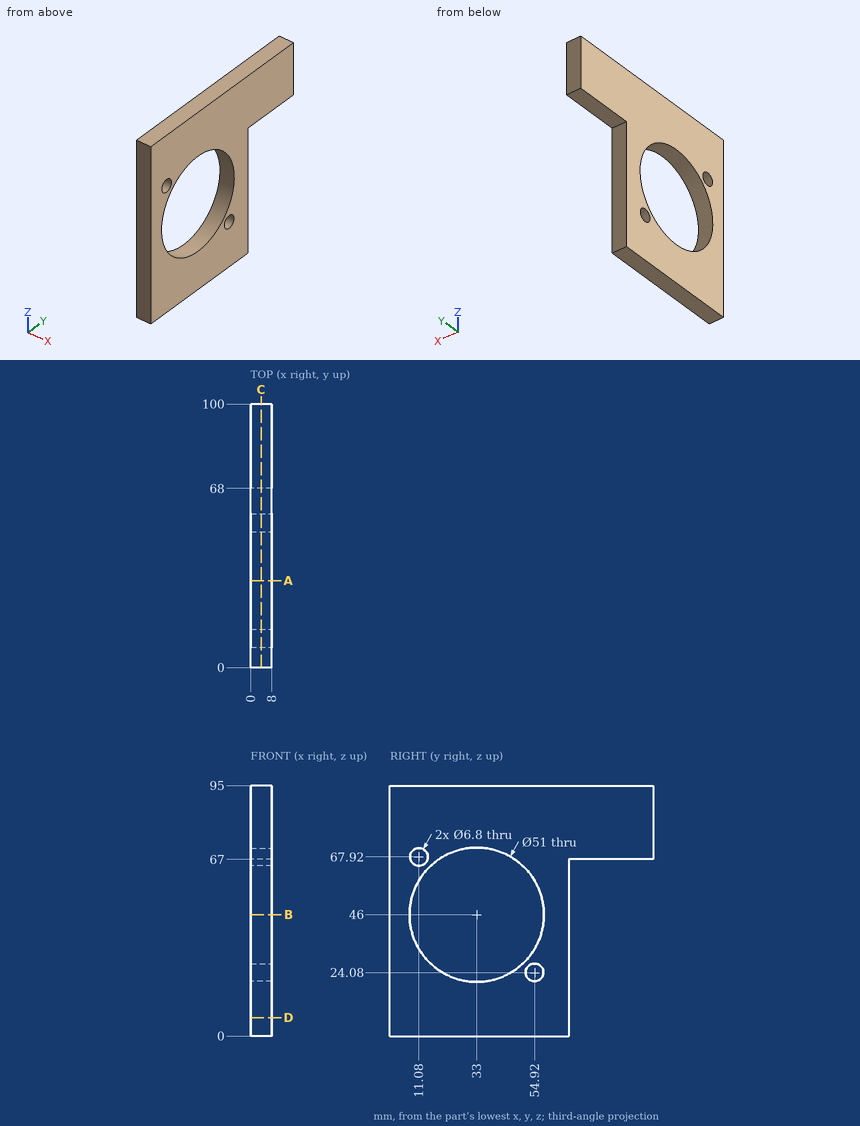
The drawing under review shows one solid part. Ordinate dimensions are in mm from its lowest x, y, z. Give positions to 0.01 mm unless a question says otherwise; leave off trailing zeros. Write each loop counter-clockwise with the first axis right and the second up, starting at its lowest first coordinate (ties: lowest second). Pieces come first, ordered by that corner, then holes. Notation, with made-up numbers: (73.25, 84.5) -> (77.25, 84.5) arc R21 ccw to (77.25, 97.5) -> close; hole circle Ø10 at (23.5, 10). An arc over 180 degrees is marked (long way). Use CSV: the item, a comma, the result in double quotes.
Q1. For P1, Ø4, axis at x = 3.5, y = 86, coming from the -Z side, flat-tipped, find the tip position at first contact; note if it passes through.
Conclusion:
P1,"z = 67"
Q2. Take a section at D-D, the plane z = 7. Write out the cut boundary in (x, y).
Conclusion:
outline,"(0, 0) -> (8, 0) -> (8, 68) -> (0, 68) -> close"
Q3. To check wall thickness, follow probe 1 along Z at (x, y) = (5.5, 55.5); probe 2 along Y at (x, z) = (2.5, 46); probe 3 along Y at (x, z) = (7.5, 27) (1 decimal). State the ranges of each line that lie inside material, in increasing order. Write a range as [from, to].
Conclusion:
probe 1,"[0, 20.73], [27.43, 34], [58, 95]"
probe 2,"[0, 7.5], [58.5, 68]"
probe 3,"[0, 16], [50, 53.2], [56.7, 68]"
Q4. Take a section at B-B, the plane z = 46. Write out the cut boundary in (x, y).
Conclusion:
outline,"(0, 0) -> (8, 0) -> (8, 7.5) -> (0, 7.5) -> close; (0, 58.5) -> (8, 58.5) -> (8, 68) -> (0, 68) -> close"
Q5. Take a section at C-C, the plane x = 4. Write out the cut boundary in (y, z).
Conclusion:
outline,"(0, 0) -> (68, 0) -> (68, 67) -> (100, 67) -> (100, 95) -> (0, 95) -> close; hole circle Ø51 at (33, 46); hole circle Ø6.8 at (11.08, 67.92); hole circle Ø6.8 at (54.92, 24.08)"
Q6. Take a section at A-A, the plane y = 33. Write out the cut boundary in (x, z), then the cut area to 3 significant figures.
Conclusion:
outline,"(0, 0) -> (8, 0) -> (8, 20.5) -> (0, 20.5) -> close; (0, 71.5) -> (8, 71.5) -> (8, 95) -> (0, 95) -> close"
area,"352 mm2"
